from build123d import *

# Parameters (mm, degrees)
BOSS_EXTRUDE1_DEPTH = 1


with BuildPart() as part:
    # Sketch1 → Boss-Extrude1 (new body)
    with BuildSketch(Plane(origin=(0, 0, 0), x_dir=(1, 0, 0), z_dir=(0, 1, 0))):
        with BuildLine():
            Line((1.85, -59.55), (3.6, -59.55))
            Line((3.6, -59.55), (3.6, 0))
            Line((3.6, 0), (1.85, 0))
            Line((1.85, 0), (1.85, -0.05))
            ThreePointArc((1.85, -0.05), (3.069759198, -0.555240802), (3.575, -1.775))
            ThreePointArc((3.575, -1.775), (3.069759198, -2.994759198), (1.85, -3.5))
            Line((1.85, -3.5), (1.85, -3.55))
            ThreePointArc((1.85, -3.55), (3.069759198, -4.055240802), (3.575, -5.275))
            ThreePointArc((3.575, -5.275), (3.069759198, -6.494759198), (1.85, -7))
            Line((1.85, -7), (1.85, -7.05))
            ThreePointArc((1.85, -7.05), (3.069759198, -7.555240802), (3.575, -8.775))
            ThreePointArc((3.575, -8.775), (3.069759198, -9.994759198), (1.85, -10.5))
            Line((1.85, -10.5), (1.85, -10.55))
            ThreePointArc((1.85, -10.55), (3.069759198, -11.055240802), (3.575, -12.275))
            ThreePointArc((3.575, -12.275), (3.069759198, -13.494759198), (1.85, -14))
            Line((1.85, -14), (1.85, -14.05))
            ThreePointArc((1.85, -14.05), (3.069759198, -14.555240802), (3.575, -15.775))
            ThreePointArc((3.575, -15.775), (3.069759198, -16.994759198), (1.85, -17.5))
            Line((1.85, -17.5), (1.85, -17.55))
            ThreePointArc((1.85, -17.55), (3.069759198, -18.055240802), (3.575, -19.275))
            ThreePointArc((3.575, -19.275), (3.069759198, -20.494759198), (1.85, -21))
            Line((1.85, -21), (1.85, -21.05))
            ThreePointArc((1.85, -21.05), (3.069759198, -21.555240802), (3.575, -22.775))
            ThreePointArc((3.575, -22.775), (3.069759198, -23.994759198), (1.85, -24.5))
            Line((1.85, -24.5), (1.85, -24.55))
            ThreePointArc((1.85, -24.55), (3.069759198, -25.055240802), (3.575, -26.275))
            ThreePointArc((3.575, -26.275), (3.069759198, -27.494759198), (1.85, -28))
            Line((1.85, -28), (1.85, -28.05))
            ThreePointArc((1.85, -28.05), (3.069759198, -28.555240802), (3.575, -29.775))
            ThreePointArc((3.575, -29.775), (3.069759198, -30.994759198), (1.85, -31.5))
            Line((1.85, -31.5), (1.85, -31.55))
            ThreePointArc((1.85, -31.55), (3.069759198, -32.055240802), (3.575, -33.275))
            ThreePointArc((3.575, -33.275), (3.069759198, -34.494759198), (1.85, -35))
            Line((1.85, -35), (1.85, -35.05))
            ThreePointArc((1.85, -35.05), (3.069759198, -35.555240802), (3.575, -36.775))
            ThreePointArc((3.575, -36.775), (3.069759198, -37.994759198), (1.85, -38.5))
            Line((1.85, -38.5), (1.85, -38.55))
            ThreePointArc((1.85, -38.55), (3.069759198, -39.055240802), (3.575, -40.275))
            ThreePointArc((3.575, -40.275), (3.069759198, -41.494759198), (1.85, -42))
            Line((1.85, -42), (1.85, -42.05))
            ThreePointArc((1.85, -42.05), (3.069759198, -42.555240802), (3.575, -43.775))
            ThreePointArc((3.575, -43.775), (3.069759198, -44.994759198), (1.85, -45.5))
            Line((1.85, -45.5), (1.85, -45.55))
            ThreePointArc((1.85, -45.55), (3.069759198, -46.055240802), (3.575, -47.275))
            ThreePointArc((3.575, -47.275), (3.069759198, -48.494759198), (1.85, -49))
            Line((1.85, -49), (1.85, -49.05))
            ThreePointArc((1.85, -49.05), (3.069759198, -49.555240802), (3.575, -50.775))
            ThreePointArc((3.575, -50.775), (3.069759198, -51.994759198), (1.85, -52.5))
            Line((1.85, -52.5), (1.85, -52.55))
            ThreePointArc((1.85, -52.55), (3.069759198, -53.055240802), (3.575, -54.275))
            ThreePointArc((3.575, -54.275), (3.069759198, -55.494759198), (1.85, -56))
            Line((1.85, -56), (1.85, -56.05))
            ThreePointArc((1.85, -56.05), (3.069759198, -56.555240802), (3.575, -57.775))
            ThreePointArc((3.575, -57.775), (3.069759198, -58.994759198), (1.85, -59.5))
            Line((1.85, -59.5), (1.85, -59.55))
        make_face()
        with BuildLine():
            Line((0, -59.55), (1.85, -59.55))
            Line((1.85, -59.55), (1.85, -59.5))
            ThreePointArc((1.85, -59.5), (0.125, -57.775), (1.85, -56.05))
            Line((1.85, -56.05), (1.85, -56))
            ThreePointArc((1.85, -56), (0.125, -54.275), (1.85, -52.55))
            Line((1.85, -52.55), (1.85, -52.5))
            ThreePointArc((1.85, -52.5), (0.125, -50.775), (1.85, -49.05))
            Line((1.85, -49.05), (1.85, -49))
            ThreePointArc((1.85, -49), (0.125, -47.275), (1.85, -45.55))
            Line((1.85, -45.55), (1.85, -45.5))
            ThreePointArc((1.85, -45.5), (0.125, -43.775), (1.85, -42.05))
            Line((1.85, -42.05), (1.85, -42))
            ThreePointArc((1.85, -42), (0.125, -40.275), (1.85, -38.55))
            Line((1.85, -38.55), (1.85, -38.5))
            ThreePointArc((1.85, -38.5), (0.125, -36.775), (1.85, -35.05))
            Line((1.85, -35.05), (1.85, -35))
            ThreePointArc((1.85, -35), (0.125, -33.275), (1.85, -31.55))
            Line((1.85, -31.55), (1.85, -31.5))
            ThreePointArc((1.85, -31.5), (0.125, -29.775), (1.85, -28.05))
            Line((1.85, -28.05), (1.85, -28))
            ThreePointArc((1.85, -28), (0.125, -26.275), (1.85, -24.55))
            Line((1.85, -24.55), (1.85, -24.5))
            ThreePointArc((1.85, -24.5), (0.125, -22.775), (1.85, -21.05))
            Line((1.85, -21.05), (1.85, -21))
            ThreePointArc((1.85, -21), (0.125, -19.275), (1.85, -17.55))
            Line((1.85, -17.55), (1.85, -17.5))
            ThreePointArc((1.85, -17.5), (0.125, -15.775), (1.85, -14.05))
            Line((1.85, -14.05), (1.85, -14))
            ThreePointArc((1.85, -14), (0.125, -12.275), (1.85, -10.55))
            Line((1.85, -10.55), (1.85, -10.5))
            ThreePointArc((1.85, -10.5), (0.125, -8.775), (1.85, -7.05))
            Line((1.85, -7.05), (1.85, -7))
            ThreePointArc((1.85, -7), (0.125, -5.275), (1.85, -3.55))
            Line((1.85, -3.55), (1.85, -3.5))
            ThreePointArc((1.85, -3.5), (0.125, -1.775), (1.85, -0.05))
            Line((1.85, -0.05), (1.85, 0))
            Line((1.85, 0), (0, 0))
            Line((0, 0), (0, -59.55))
        make_face()
        with BuildLine():
            Line((5.35, -59.5), (5.35, -59.55))
            Line((5.35, -59.55), (7.2, -59.55))
            Line((7.2, -59.55), (7.2, 0))
            Line((7.2, 0), (5.35, 0))
            Line((5.35, 0), (5.35, -0.05))
            ThreePointArc((5.35, -0.05), (6.569759198, -0.555240802), (7.075, -1.775))
            ThreePointArc((7.075, -1.775), (6.569759198, -2.994759198), (5.35, -3.5))
            Line((5.35, -3.5), (5.35, -3.55))
            ThreePointArc((5.35, -3.55), (6.569759198, -4.055240802), (7.075, -5.275))
            ThreePointArc((7.075, -5.275), (6.569759198, -6.494759198), (5.35, -7))
            Line((5.35, -7), (5.35, -7.05))
            ThreePointArc((5.35, -7.05), (6.569759198, -7.555240802), (7.075, -8.775))
            ThreePointArc((7.075, -8.775), (6.569759198, -9.994759198), (5.35, -10.5))
            Line((5.35, -10.5), (5.35, -10.55))
            ThreePointArc((5.35, -10.55), (6.569759198, -11.055240802), (7.075, -12.275))
            ThreePointArc((7.075, -12.275), (6.569759198, -13.494759198), (5.35, -14))
            Line((5.35, -14), (5.35, -14.05))
            ThreePointArc((5.35, -14.05), (6.569759198, -14.555240802), (7.075, -15.775))
            ThreePointArc((7.075, -15.775), (6.569759198, -16.994759198), (5.35, -17.5))
            Line((5.35, -17.5), (5.35, -17.55))
            ThreePointArc((5.35, -17.55), (6.569759198, -18.055240802), (7.075, -19.275))
            ThreePointArc((7.075, -19.275), (6.569759198, -20.494759198), (5.35, -21))
            Line((5.35, -21), (5.35, -21.05))
            ThreePointArc((5.35, -21.05), (6.569759198, -21.555240802), (7.075, -22.775))
            ThreePointArc((7.075, -22.775), (6.569759198, -23.994759198), (5.35, -24.5))
            Line((5.35, -24.5), (5.35, -24.55))
            ThreePointArc((5.35, -24.55), (6.569759198, -25.055240802), (7.075, -26.275))
            ThreePointArc((7.075, -26.275), (6.569759198, -27.494759198), (5.35, -28))
            Line((5.35, -28), (5.35, -28.05))
            ThreePointArc((5.35, -28.05), (6.569759198, -28.555240802), (7.075, -29.775))
            ThreePointArc((7.075, -29.775), (6.569759198, -30.994759198), (5.35, -31.5))
            Line((5.35, -31.5), (5.35, -31.55))
            ThreePointArc((5.35, -31.55), (6.569759198, -32.055240802), (7.075, -33.275))
            ThreePointArc((7.075, -33.275), (6.569759198, -34.494759198), (5.35, -35))
            Line((5.35, -35), (5.35, -35.05))
            ThreePointArc((5.35, -35.05), (6.569759198, -35.555240802), (7.075, -36.775))
            ThreePointArc((7.075, -36.775), (6.569759198, -37.994759198), (5.35, -38.5))
            Line((5.35, -38.5), (5.35, -38.55))
            ThreePointArc((5.35, -38.55), (6.569759198, -39.055240802), (7.075, -40.275))
            ThreePointArc((7.075, -40.275), (6.569759198, -41.494759198), (5.35, -42))
            Line((5.35, -42), (5.35, -42.05))
            ThreePointArc((5.35, -42.05), (6.569759198, -42.555240802), (7.075, -43.775))
            ThreePointArc((7.075, -43.775), (6.569759198, -44.994759198), (5.35, -45.5))
            Line((5.35, -45.5), (5.35, -45.55))
            ThreePointArc((5.35, -45.55), (6.569759198, -46.055240802), (7.075, -47.275))
            ThreePointArc((7.075, -47.275), (6.569759198, -48.494759198), (5.35, -49))
            Line((5.35, -49), (5.35, -49.05))
            ThreePointArc((5.35, -49.05), (6.569759198, -49.555240802), (7.075, -50.775))
            ThreePointArc((7.075, -50.775), (6.569759198, -51.994759198), (5.35, -52.5))
            Line((5.35, -52.5), (5.35, -52.55))
            ThreePointArc((5.35, -52.55), (6.569759198, -53.055240802), (7.075, -54.275))
            ThreePointArc((7.075, -54.275), (6.569759198, -55.494759198), (5.35, -56))
            Line((5.35, -56), (5.35, -56.05))
            ThreePointArc((5.35, -56.05), (6.569759198, -56.555240802), (7.075, -57.775))
            ThreePointArc((7.075, -57.775), (6.569759198, -58.994759198), (5.35, -59.5))
        make_face()
        with BuildLine():
            Line((3.6, 0), (3.6, -59.55))
            Line((3.6, -59.55), (5.35, -59.55))
            Line((5.35, -59.55), (5.35, -59.5))
            ThreePointArc((5.35, -59.5), (3.625, -57.775), (5.35, -56.05))
            Line((5.35, -56.05), (5.35, -56))
            ThreePointArc((5.35, -56), (3.625, -54.275), (5.35, -52.55))
            Line((5.35, -52.55), (5.35, -52.5))
            ThreePointArc((5.35, -52.5), (3.625, -50.775), (5.35, -49.05))
            Line((5.35, -49.05), (5.35, -49))
            ThreePointArc((5.35, -49), (3.625, -47.275), (5.35, -45.55))
            Line((5.35, -45.55), (5.35, -45.5))
            ThreePointArc((5.35, -45.5), (3.625, -43.775), (5.35, -42.05))
            Line((5.35, -42.05), (5.35, -42))
            ThreePointArc((5.35, -42), (3.625, -40.275), (5.35, -38.55))
            Line((5.35, -38.55), (5.35, -38.5))
            ThreePointArc((5.35, -38.5), (3.625, -36.775), (5.35, -35.05))
            Line((5.35, -35.05), (5.35, -35))
            ThreePointArc((5.35, -35), (3.625, -33.275), (5.35, -31.55))
            Line((5.35, -31.55), (5.35, -31.5))
            ThreePointArc((5.35, -31.5), (3.625, -29.775), (5.35, -28.05))
            Line((5.35, -28.05), (5.35, -28))
            ThreePointArc((5.35, -28), (3.625, -26.275), (5.35, -24.55))
            Line((5.35, -24.55), (5.35, -24.5))
            ThreePointArc((5.35, -24.5), (3.625, -22.775), (5.35, -21.05))
            Line((5.35, -21.05), (5.35, -21))
            ThreePointArc((5.35, -21), (3.625, -19.275), (5.35, -17.55))
            Line((5.35, -17.55), (5.35, -17.5))
            ThreePointArc((5.35, -17.5), (3.625, -15.775), (5.35, -14.05))
            Line((5.35, -14.05), (5.35, -14))
            ThreePointArc((5.35, -14), (3.625, -12.275), (5.35, -10.55))
            Line((5.35, -10.55), (5.35, -10.5))
            ThreePointArc((5.35, -10.5), (3.625, -8.775), (5.35, -7.05))
            Line((5.35, -7.05), (5.35, -7))
            ThreePointArc((5.35, -7), (3.625, -5.275), (5.35, -3.55))
            Line((5.35, -3.55), (5.35, -3.5))
            ThreePointArc((5.35, -3.5), (3.625, -1.775), (5.35, -0.05))
            Line((5.35, -0.05), (5.35, 0))
            Line((5.35, 0), (3.6, 0))
        make_face()
    extrude(amount=BOSS_EXTRUDE1_DEPTH)


solid = part.part
Model file for the job. Use its own axes, mm. Round coordinates to 2 decimals unless told otherwise and drop trailing zeros. Order: outer loops, then holes, each group sorted by start corner. A loop starts at its lowest first (then second) coordinate and runs counter-clockwise, first axis right, second up.
(1) Band-saw the part on B-B (x = 4.5). Give the number of separate pieces and of enclosed holes in the cut face, then the cut area to 3 significant figures.
(2) Drill centre lines: line 1 (X direction, y = 0.65, z = 11); line 2 (X direction, y = 0.7, z = 36). Where is each one in solid material? Low to high.
(3) Band-saw the part on A-A (z = 30.5). List the corners of the cut face in (x, y), then the cut area to 3 significant figures.
Verdict:
1. separate pieces: 18
1. enclosed holes: 0
1. area: 8.51 mm2
2. line 1: x = 0 to 0.69, 3.01 to 4.19, 6.51 to 7.2
2. line 2: x = 0 to 0.31, 3.39 to 3.81, 6.89 to 7.2
3. outline: (0, 0) - (0.28, 0) - (0.28, 1) - (0, 1) - close; (3.42, 0) - (3.78, 0) - (3.78, 1) - (3.42, 1) - close; (6.92, 0) - (7.2, 0) - (7.2, 1) - (6.92, 1) - close
3. area: 0.939 mm2
